Part model, mm, in its own coordinate system. Face numbers are marked on the shaded views. A direction names the side the tool comes from. Give positions to 0.01 mm unless a question says otherwise; leave off trailing zeros. Write each loop counter-clockwise with the first axis right and the second up, starting at its lowest first coordinate (ties: lowest second). Pieces come first, ordered by that corner, then holes. Notation, with made-up numbers: M 4,1.25 L 32,1.25 A12 cw 32,11.25 Z; hole C 73,47.5 d10. An arc over 180 degrees is marked long. Use CSV: the item, a comma, the result in double quotes. Start each with the question number.
1. Band-saw the part on A-A, the plane z = 5.5. List the corners of the cut face in (x, y) (3 decimals).
2. Band-saw the part on B-B, the plane x = 12.25. List the corners of the cut face in (y, z), then the cut area to 3 significant figures.
3. Drop flat-ended pins along their axis: pin 1 Ø3 at (x, z) = (-3.5, 9) entering from +Y; pin 2 Ø1 at (x, y) = (-3, 21.5) entering from -Z; pin 3 Ø5 at (y, z) = (-1, 3.5) entering from +X; pin 4 Ø3 at (y, z) = (-1.5, 6) entering from -X. Give the stop position or say it passes through.
4. 3-axis set-ups, long thin cutter, end or side, ignore diameter. For the marked faces 1, 2 and 3: which of +Z, -Z, +X, -X, +Y, -Y reach the whole face in a straight line?
5. Drill centre lines: line 1 along X through (y, z) = (2, 6); line 2 along Y through (x, z) = (7.75, 7.5) (3 decimals); line 3 along Y through (x, z) = (8, 10) (3 decimals). Where is each one in solid material? Low to high. Write a range as from..to.
from build123d import *

# Parameters (mm, degrees)
BOSS_EXTRUDE1_DEPTH = 12.29


with BuildPart() as part:
    # Sketch2 → Boss-Extrude1 (new body)
    with BuildSketch(Plane.XY):
        with BuildLine():
            Line((-8.74, 3.175), (-7.47, 3.175))
            Line((-7.47, 3.175), (-7.47, 3.937))
            Line((-7.47, 3.937), (-8.232, 3.937))
            ThreePointArc((-8.232, 3.937), (0, 29.470311879), (8.232, 3.937))
            Line((8.232, 3.937), (7.47, 3.937))
            Line((7.47, 3.937), (7.47, 3.175))
            Line((7.47, 3.175), (8.74, 3.175))
            Line((8.74, 3.175), (8.74, -3.175))
            Line((8.74, -3.175), (-8.74, -3.175))
            Line((-8.74, -3.175), (-8.74, 3.175))
        make_face()
    extrude(amount=BOSS_EXTRUDE1_DEPTH)


solid = part.part
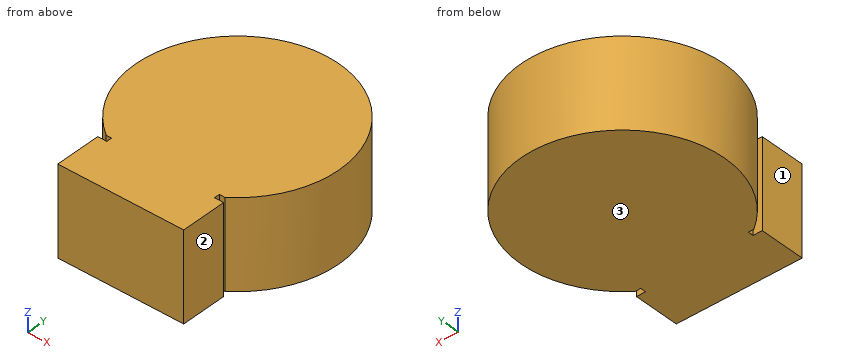
Output:
1,outline,"M -8.74,-3.175 L 8.74,-3.175 L 8.74,3.175 L 7.47,3.175 L 7.47,3.937 L 8.232,3.937 A14.094 ccw long -8.232,3.937 L -7.47,3.937 L -7.47,3.175 L -8.74,3.175 Z"
2,outline,"M 8.41,0 L 22.35,0 L 22.35,12.29 L 8.41,12.29 Z"
2,area,"171 mm²"
3,pin 1,"stops at y = 29.33"
3,pin 2,"stops at z = 0"
3,pin 3,"stops at x = 8.74"
3,pin 4,"stops at x = -8.74"
4,face 1,"+Z, -Z, -X, -Y"
4,face 2,"+Z, -Z, +X, -Y"
4,face 3,"-Z, +X, -X, +Y, -Y"
5,line 1,"x = -8.74..8.74"
5,line 2,"y = -3.175..3.175, 3.937..27.148"
5,line 3,"y = -3.175..3.175, 3.937..26.98"
